The drawing under review shows one solid part. Ordinate dimensions are in mm from its lowest x, y, z. A direction names the side the tool comes from. Round coordinates to 2 decimals unless told otherwise and drop trailing zeros. Order: outer loops, then holes, each group sorted by start corner. A loop starts at its lowest first (then second) coordinate and runs counter-clockwise, first axis right, second up. Notation, with made-up numbers: M 50,84.5 L 74,84.5 A28 cw 74,115.5 Z; hole C -13.75,9 d9. An arc over 180 degrees is marked long. Answer as a JSON object with one key per item and string values. Group by question number.
1. Mouldability with a two-part tool opening along X and no side actions: class the marked faces 1, 2 and 3 as released by +X, released by -X, zero draft, split by the parting line, or undercut.
2. To check wall thickness, follow probe 1 along Y at (x, z) = (2.5, 5.05); probe 2 along X at (y, z) = (16.25, 2); probe 3 along Z at (x, y) = (11.75, 11.75). State the ranges of each line that lie inside material, in increasing order. Write a range as [from, to].
3. Clearance check with flat-ended pins moving along their axes: P1, Ø1.6, axis at x = 14.5, y = 7.25, coming from the +Z side; P2, Ø4, axis at x = 8.5, y = 14, coming from the -Z side. State where each tip first meets the part, or that it passes through.
4. Add section C-C on z = 4.5. State the section outline as (x, y) points.
5. Machinability: for the marked faces 4 and 5, which of the approach directions +Z, -Z, +X, -X, +Y, -Y give a long, thin tool a straight path to every point of the face, cutting with its end or side? Answer none if there is none.
6. Add section B-B on x = 14.5. State the section outline as (y, z) points, and give its area (3 significant figures).
7. Add section D-D on y = 15.25. State the section outline as (x, z) points.
8. Add section A-A on y = 9.5. State the section outline as (x, z) points.
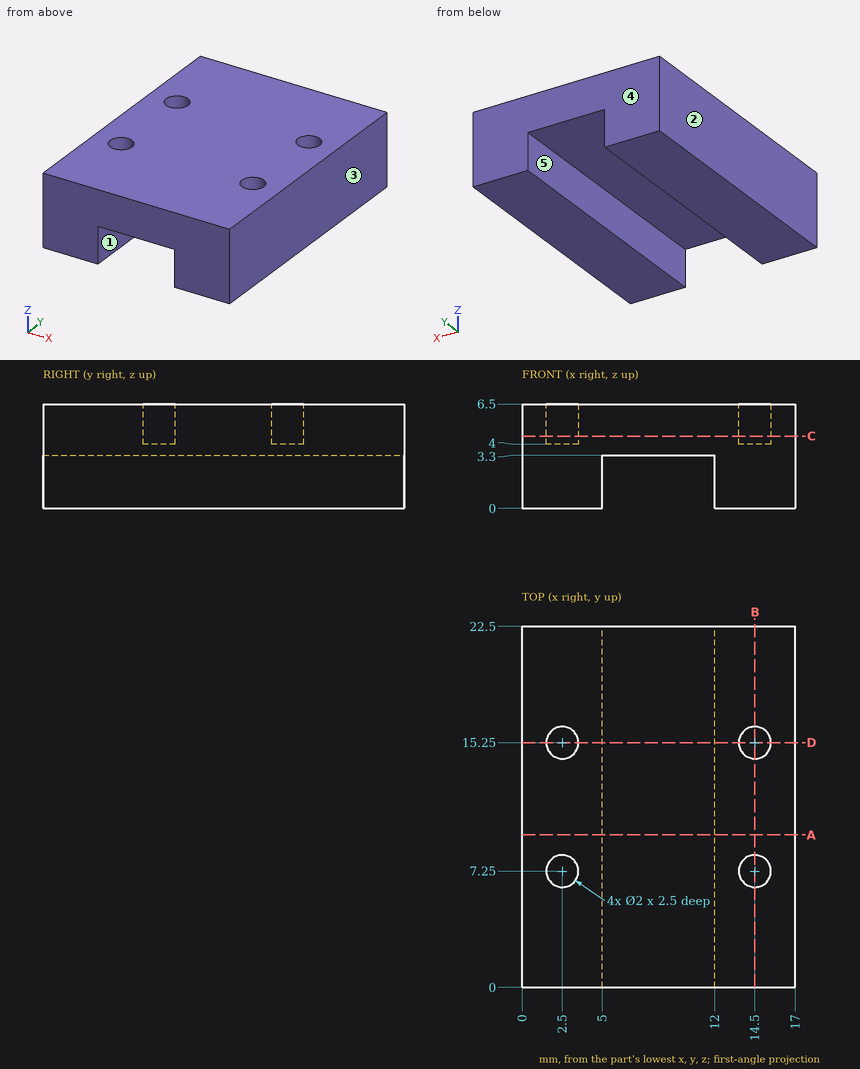
Recorded:
{
 "1": {"face 1": "undercut", "face 2": "released by -X", "face 3": "released by +X"},
 "2": {"probe 1": "y = [0, 6.25], [8.25, 14.25], [16.25, 22.5]", "probe 2": "x = [0, 5], [12, 17]", "probe 3": "z = [3.3, 6.5]"},
 "3": {"P1": "stops at z = 4", "P2": "stops at z = 3.3"},
 "4": {"outline": "M 0,0 L 17,0 L 17,22.5 L 0,22.5 Z; hole C 2.5,7.25 d2; hole C 2.5,15.25 d2; hole C 14.5,7.25 d2; hole C 14.5,15.25 d2"},
 "5": {"face 4": "+Z, -Z, +X, -X, +Y", "face 5": "-Z, +Y, -Y"},
 "6": {"outline": "M 0,0 L 22.5,0 L 22.5,6.5 L 16.25,6.5 L 16.25,4 L 14.25,4 L 14.25,6.5 L 8.25,6.5 L 8.25,4 L 6.25,4 L 6.25,6.5 L 0,6.5 Z", "area": "136 mm²"},
 "7": {"outline": "M 0,0 L 5,0 L 5,3.3 L 12,3.3 L 12,0 L 17,0 L 17,6.5 L 15.5,6.5 L 15.5,4 L 13.5,4 L 13.5,6.5 L 3.5,6.5 L 3.5,4 L 1.5,4 L 1.5,6.5 L 0,6.5 Z"},
 "8": {"outline": "M 0,0 L 5,0 L 5,3.3 L 12,3.3 L 12,0 L 17,0 L 17,6.5 L 0,6.5 Z"}
}
